from build123d import *

# Parameters (mm, degrees)
SKETCH3_R          = 13.890625
SKETCH3_R_2        = 7.8994
SKETCH4_R          = 10.795
CUT_EXTRUDE1_DEPTH = 19.05
SKETCH5_R          = 10.795
CUT_EXTRUDE2_DEPTH = 19.05


with BuildPart() as part:
    # Sweep1: sweep along a path in Sketch2
    with BuildLine(Plane(origin=(0, 0, 0), x_dir=(0, 0, -1), z_dir=(1, 0, 0))) as sweep1_path:
        Line((-17.960512242, -17.960512242), (-4.490128061, -4.490128061))
        ThreePointArc((-4.490128061, -4.490128061), (-1.166946263, 0.483364969), (0, 6.35))
        Line((0, 6.35), (0, 25.4))
    # Sketch3 → Sweep1 (sweep)
    with BuildSketch(Plane(origin=(0, 25.4, 0), x_dir=(1, 0, 0), z_dir=(0, 1, 0))):
        Circle(SKETCH3_R)
        Circle(SKETCH3_R_2, mode=Mode.SUBTRACT)
    sweep(path=sweep1_path.line)

    # Sketch4 → Cut-Extrude1 (cut)
    with BuildSketch(Plane(origin=(0, 25.4, 0), x_dir=(1, 0, 0), z_dir=(0, 1, 0))):
        with Locations(Location((0, 0, 0), (0, 0, 270))):
            Circle(SKETCH4_R)
    extrude(amount=-CUT_EXTRUDE1_DEPTH, mode=Mode.SUBTRACT)

    # Sketch5 → Cut-Extrude2 (cut)
    with BuildSketch(Plane(origin=(0, -17.960512242, 17.960512242), x_dir=(1, 0, 0), z_dir=(0, -0.7071067811865559, 0.7071067811865392))):
        with Locations(Location((0, 0, 0), (0, 0, 270))):
            Circle(SKETCH5_R)
    extrude(amount=-CUT_EXTRUDE2_DEPTH, mode=Mode.SUBTRACT)


solid = part.part
Design review of the part built by this model. Coordinates are the model's own, in mm. A direction names the side the tool comes from. Coordinates: 2 decimals unless noted, no trailing zeros. Write each loop counter-clockwise with the first axis right and the second up, starting at its lowest first coordinate (ties: lowest second). Pieces come first, ordered by that corner, then holes. Notation, with made-up numbers: (-29.75, 3.25) - (4.25, 3.25) arc R14 ccw to (4.25, 12.25) - close; hole circle Ø3 at (-2.75, 7). An arc over 180 degrees is marked (long way). Use one line per item in the form item = value.
Q1. Consider section B-B (y = 22). Write out the cut boundary in (x, z) (3 decimals), plus the area to 3 significant figures.
Taken from the geometry:
outline = circle Ø27.781 at (0, 0); hole circle Ø21.59 at (0, 0)
area = 240 mm^2
Q2. For probe 1 along X at (y, z) = (-5, 1); probe 2 along X at (y, z) = (-16, 13.5); probe 3 along Z at (x, y) = (-1.5, 4), list the stretches that pass through material, from the lowest coordinate up.
Taken from the geometry:
probe_1 = -13.57 to -7.33, 7.33 to 13.57
probe_2 = -13.78 to -10.65, 10.65 to 13.78
probe_3 = -13.71 to -7.64, 8.13 to 15.53
Q3. The part is to be moulded in two halves that separate along Z. For faces 4 (the cylindrical face through (7.296, 16.008, -7.956)), 5 (the cylindrical face through (-1.808, -20.87, 1.392)), 6 (the cylindrical face through (-4.135, -18.371, 4.268)), 7 (the flat face through (-7.14, 25.4, -8.3)), say which applies: +Z half, -Z half, draft (parallel to the pull), parting line (faces both ways), or undercut.
Taken from the geometry:
face_4 = undercut
face_5 = parting line
face_6 = undercut
face_7 = draft
Q4. Consider section A-A (x = 3). Write out the cut boundary in (y, z).
Taken from the geometry:
outline = (-27.55, 8.37) - (-14.08, -5.1) arc R28.89 ccw to (6.35, -13.56) - (25.4, -13.56) - (25.4, -10.37) - (6.35, -10.37) - (6.35, -7.31) arc R22.64 cw to (-9.66, -0.68) - (-11.82, -2.84) - (-25.29, 10.63) - close; (-10.63, 25.29) - (2.84, 11.82) - (0.68, 9.66) arc R8.02 ccw to (6.35, 7.31) - (6.35, 10.37) - (25.4, 10.37) - (25.4, 13.56) - (6.35, 13.56) arc R1.77 cw to (5.1, 14.08) - (-8.37, 27.55) - close
Q5. Consider section D-D (x = 0). Write out the cut boundary in (y, z) (3 decimals).
Taken from the geometry:
outline = (-27.783, 8.138) - (-14.312, -5.332) arc R29.221 ccw to (6.35, -13.891) - (25.4, -13.891) - (25.4, -10.795) - (6.35, -10.795) - (6.35, -7.899) arc R23.23 cw to (-10.076, -1.096) - (-12.123, -3.143) - (-25.594, 10.327) - close; (-10.327, 25.594) - (3.143, 12.123) - (1.096, 10.076) arc R7.431 ccw to (6.35, 7.899) - (6.35, 10.795) - (25.4, 10.795) - (25.4, 13.891) - (6.35, 13.891) arc R1.44 cw to (5.332, 14.312) - (-8.138, 27.783) - close
Q6. Insertion check: pin 1 Ø4 at (x, z) = (-10.5, -1) entering from -Y; pin 2 Ø4 at (x, y) = (-5.5, -9) entering from -Z; pin 3 Ø4 at (y, z) = (6, 7) entering from -X. Each pin has a flat end and moves straight along its axis. Give the tip position at first contact, or say it passes through.
Taken from the geometry:
pin_1 = -15.29
pin_2 = -9.68
pin_3 = -12.96
Q7. Machinability: for faces 1 (the cylindrical face through (-1.808, 16.008, -13.772)), 2 (the flat face through (-7.95, -3.32, 5.66)), 3 (the flat face through (7.14, -12.09, 23.83)), which of the approach directions +Z, -Z, +X, -X, +Y, -Y give a long, thin tool a straight path to every point of the face, cutting with its end or side? Answer none if there is none.
Taken from the geometry:
face_1 = +Y
face_2 = none
face_3 = +Z, +X, -X, -Y
Q8. Consider section C-C (x = -9.5). Write out the cut boundary in (y, z), plus the area to 3 significant figures.
Taken from the geometry:
outline = (-25.13, 10.79) - (-11.66, -2.68) arc R25.46 ccw to (6.35, -10.13) - (25.4, -10.13) - (25.4, -5.13) - (6.35, -5.13) - (6.35, 5.13) - (25.4, 5.13) - (25.4, 10.13) - (6.35, 10.13) arc R5.2 cw to (2.68, 11.66) - (-10.79, 25.13) - (-14.34, 21.59) - (-0.87, 8.12) - (-8.12, 0.87) - (-21.59, 14.34) - close
area = 626 mm^2
